from build123d import *

# Parameters (mm, degrees)
F0_W     = 19.05
F0_H     = 6.35
F1_DEPTH = 25.4
F2_START = -6.35
F2_DEPTH = 19.05
F4_W     = 19.05
F4_H     = 6.35
F5_DEPTH = 38.101
F6_R     = 3.175
F7_DEPTH = 31.751


with BuildPart() as f1:
    # F0 (on Front) → F1 (new body)
    with BuildSketch(Plane.XZ):
        with Locations((28.575, 28.575)):
            Rectangle(F0_W, F0_H)
        Polygon((19.05, 25.4), (19.05, 12.7), (19.05, 6.35), (38.1, 6.35), (38.1, 25.4), align=None)
    extrude(amount=-F1_DEPTH)

    # F0 (on Front) → F2 (join)
    with BuildSketch(Plane.XZ.offset(F2_START)):
        Polygon((0, 12.7), (0, 0), (6.35, 0), (6.35, 6.35), (19.05, 6.35), (19.05, 12.7), align=None)
    extrude(amount=-F2_DEPTH)

    # F4 (on face) → F5 (cut, through all)
    with BuildSketch(Plane.YZ.offset(38.1)):
        with Locations((9.525, 28.575)):
            Rectangle(F4_W, F4_H)
    extrude(amount=-F5_DEPTH, mode=Mode.SUBTRACT)

    # F6 (on Top) → F7 (cut, through all)
    with BuildSketch(Plane.XY):
        with Locations((12.7, 15.875)):
            Circle(F6_R)
        with Locations((28.575, 9.525)):
            Circle(F6_R)
    extrude(amount=F7_DEPTH, mode=Mode.SUBTRACT)


solid = f1.part
Input: part model. Units: mm. Frame: model coordinates. A direction names the side the tool comes from. Give positions to 0.01 mm unless a question says otherwise; leave off trailing zeros. Order: outer loops, then holes, each group sorted by start corner. A loop starts at its lowest first (then second) coordinate and runs counter-clockwise, first axis right, second up. Notation, with made-up numbers: (75.5, -9.5) - (123.5, -9.5) arc R29 ccw to (123.5, 12.5) - close; hole circle Ø4 at (-11, 13). An arc over 180 degrees is marked (long way). Answer as a JSON object with one key per item and string values. Group by question number.
Q1. Line query: probe 1 along Y at (x, z) = (28.5, 11.5); probe 2 along X at (y, z) = (16.5, 21); probe 3 along X at (y, z) = (9, 6). Output: solid intervals per line, ascending.
Q2. Cut plane C-C, the plane y = 20.25. Output: boundary loops of the cut face in (x, z).
Q3. Cut plane B-B, the plane x = 12.7. Output: boundary loops of the cut face in (y, z), then the cut area to 3 significant figures.
Q4. First-contact query: pin 1 Ø6.5 at (x, z) = (9.5, 8.5) entering from -Y; pin 2 Ø1.5 at (x, y) = (21, 7) entering from +Z; pin 3 Ø5.5 at (x, y) = (12.7, 15.875) entering from -Z; pin 4 Ø5 at (x, z) = (29.5, 28.5) entering from -Y. Flat tips, straight axial feed; report the tip coordinate or a pass-through.
Q5. Cut plane A-A, the plane z = 8. Output: boundary loops of the cut face in (x, y) (3 decimals).
Q6. Mould query, pull axis X, two halves, no side actions, for faces 1 (the face through (8, 16, 12.7)), 2 (the face through (0, 16, 6)), 3 (the face through (26.235, 11.671, 15.742)). Classes: pulls with the +X half, pulls with the -X half, needs draft (parallel to the pull), parting line crosses it, or undercut.
Q7. Cut plane D-D, the plane y = 10.5. Output: boundary loops of the cut face in (x, z).
Q8. Set-up query: faces 4 (the face through (31, 7, 25.4)), 5 (the face through (7, 6.35, 8)), 6 (the face through (28, 0, 16)), 7 (the face through (6.35, 16, 3)). Return all of +Z, -Z, +X, -X, +Y, -Y with unobstructed straight access to the full face (end or side cutting, diameter ignored); none if empty.
Results:
{
 "1": {"probe 1": "0 to 6.35, 12.7 to 25.4", "probe 2": "19.05 to 38.1", "probe 3": "0 to 6.35"},
 "2": {"outline": "(0, 0) - (6.35, 0) - (6.35, 6.35) - (38.1, 6.35) - (38.1, 31.75) - (19.05, 31.75) - (19.05, 12.7) - (0, 12.7) - close"},
 "3": {"outline": "(6.35, 6.35) - (12.7, 6.35) - (12.7, 12.7) - (6.35, 12.7) - close; (19.05, 6.35) - (25.4, 6.35) - (25.4, 12.7) - (19.05, 12.7) - close", "area": "80.6 mm^2"},
 "4": {"pin 1": "y = 6.35", "pin 2": "z = 25.4", "pin 3": "through", "pin 4": "y = 19.05"},
 "5": {"outline": "(0, 6.35) - (19.05, 6.35) - (19.05, 0) - (38.1, 0) - (38.1, 25.4) - (0, 25.4) - close; hole circle Ø6.35 at (12.7, 15.875); hole circle Ø6.35 at (28.575, 9.525)"},
 "6": {"face 1": "needs draft", "face 2": "pulls with the -X half", "face 3": "undercut"},
 "7": {"outline": "(0, 0) - (6.35, 0) - (6.35, 6.35) - (25.55, 6.35) - (25.55, 25.4) - (19.05, 25.4) - (19.05, 12.7) - (0, 12.7) - close; (31.6, 6.35) - (38.1, 6.35) - (38.1, 25.4) - (31.6, 25.4) - close"},
 "8": {"face 4": "+Z, +X, -X, -Y", "face 5": "+Z, -Z, -X, -Y", "face 6": "+Z, -Z, +X, -X, -Y", "face 7": "-Z, +X, +Y, -Y"}
}
